Autodesk Inventor part; units mm, degrees
ref_plane "Work Plane1" through (0, 5, 0) normal (0, 1, 0) x (-1, 0, 0)
ref_plane "YZ Plane" through (0, 0, 0) normal (1, 0, 0) x (0, 1, 0)
ref_plane "XY Plane" through (0, 0, 0) normal (0, 0, 1) x (1, 0, 0)
sketch "Sketch1" plane through (0, 0, 0) normal (1, 0, 0) x (0, 1, 0)
  circle A0 centre (0, 0) radius 3.625
  circle A1 centre (0, 0) radius 5
  dimension "d0" = 7.25
  dimension "d1" = 10
extrude "Extrusion1" add sketch "Sketch1" along normal mid plane 20
ref_plane "Work Plane1" through (0, 5, 0) normal (0, 1, 0) x (-1, 0, 0)
sketch "Sketch2" plane through (0, 5, 0) normal (0, 1, 0) x (-1, 0, 0)
  line L0 (-1.65, 2.15) -> (1.65, 2.15)
  line L1 (1.65, 2.15) -> (1.65, -2.15)
  line L2 (1.65, -2.15) -> (-1.65, -2.15)
  line L3 (-1.65, -2.15) -> (-1.65, 2.15)
  line L4 (-1.65, 2.15) -> (1.65, -2.15) construction
  line L5 (1.65, 2.15) -> (-1.65, -2.15) construction
  line L6 (-4, 3) -> (4, 3)
  line L7 (4, 3) -> (4, -3)
  line L8 (4, -3) -> (-4, -3)
  line L9 (-4, -3) -> (-4, 3)
  line L10 (-4, 3) -> (4, -3) construction
  line L11 (4, 3) -> (-4, -3) construction
  arc A0 (1.65, -2.15) -> (1.65, 2.15) centre (0.0168, 0) ccw
  arc A1 (-1.65, 2.15) -> (-1.65, -2.15) centre (-0.0168, 0) ccw
  point P0 (0, 0)
  dimension "d4" = 3.3
  dimension "d5" = 4.3
  dimension "d9" = 8
  dimension "d10" = 6
  dimension "d15" = 2.7
  dimension "d16" = 2.7
extrude "Extrusion2" add sketch "Sketch2" against normal blind 4.125 contours L0 L1 L2 L3 | L3 A1 | A0 L1 | L6 L7 L8 L9
extrude "Extrusion3" cut sketch "Sketch2" against normal up to surface (4.125 mm away) contours L0 L1 L2 L3 | L3 A1 | A0 L1
ref_plane "Work Plane2" through (0, -5, 0) normal (0, 1, 0) x (-1, 0, 0)
sketch "Sketch3" plane through (0, -5, 0) normal (0, 1, 0) x (-1, 0, 0)
  line L0 (10, 3.625) -> (10, -3.625)
  line L1 (-10, 5) -> (-10, -5)
  line L2 (10, 2) -> (-10, 2)
  line L3 (-10, 2) -> (-10, -2)
  line L4 (-10, -2) -> (10, -2)
  line L5 (10, -2) -> (10, 2)
  point P0 (0, 0)
  point P1 (0, 2)
  dimension "d17" = 4
  dimension "d18" = 2
extrude "Extrusion4" add sketch "Sketch3" along normal blind 1
properties part number "part_holder"
The model under review builds one solid part; all positions refer to its coordinate system, in mm. A direction names the side the tool comes from. Round coordinates to 2 decimals unless told otherwise and drop trailing zeros. Order: outer loops, then holes, each group sorted by start corner. A loop starts at its lowest first (then second) coordinate and runs counter-clockwise, first axis right, second up. Notation, with made-up numbers: (82, 62) -> (120, 62) arc R21 cw to (120, 92) -> close; hole circle Ø5 at (0.25, 43). An arc over 180 degrees is marked (long way). Write item = value, one per line. Start each with the question number.
Item 1: Consider section A-A on y = 0. Write out the cut boundary in (x, z) (3 decimals), plus the area to 3 significant figures.
Item 2: Consider section C-C on x = 1.25. Write out the cut boundary in (y, z) (3 decimals).
Item 3: For line 1 along Z through (x, y) = (0, 0) (3 decimals); line 2 along Y through (x, z) = (-6.75, 4); line 3 along Z through (x, y) = (-7, -1.5), list the stretches that pass through material, from the lowest coordinate up.
Item 4: Mouldability with a two-part tool opening along Y and no side actions: class faces 4 (the face through (-0.14, 1.569, 4.747)), 5 (the face through (-4, 4.7, -2.3)), 6 (the face through (4, 2, 0)) as released by +Y, released by -Y, zero draft, split by the parting line, or undercut.
Item 5: Consider section D-D on y = -3. Write out the cut boundary in (x, z), plus the area to 3 significant figures.
Item 6: Clearance check with flat-ended pins moving along their axes: pin 1 Ø0.5 at (x, y) = (-1.5, 4.5) entering from -Z; pin 2 Ø2 at (x, y) = (6.5, 1.5) entering from +Z; pin 3 Ø6 at (y, z) = (0, 0) entering from +X. State where each tip first meets the part, or that it passes through.
Item 7: For faces 1 (the face through (4, 4.7, 2.3)), 2 (the face through (0, 3, 2.15)), 3 (the face through (-0.1, 4.5, -3)), list the 3-axis set-ups (+Z, -Z, +X, -X, +Y, -Y) from which the entire face can be reached by the end or side of a thin tool; tool diameter is ignored.
Item 8: Consider section B-B on x = 7.25. Write out the cut boundary in (y, z) (3 decimals), plus the area to 3 significant figures.
Conclusion:
q1.outline = (-10, -5) -> (10, -5) -> (10, -3.625) -> (-10, -3.625) -> close; (-10, 3.625) -> (10, 3.625) -> (10, 5) -> (-10, 5) -> close
q1.area = 55.0 mm2
q2.outline = (-5, -2) -> (-4.583, -2) arc R5 ccw to (4, -3) -> (5, -3) -> (5, -2.15) -> (0.875, -2.15) -> (0.875, -3) -> (2.035, -3) arc R3.625 cw (long way) to (2.035, 3) -> (0.875, 3) -> (0.875, 2.15) -> (5, 2.15) -> (5, 3) -> (4, 3) arc R5 ccw to (-4.583, 2) -> (-5, 2) -> close
q3.line_1 = -5 to -3.625, 3.625 to 5
q3.line_2 = -3 to 3
q3.line_3 = -4.77 to -3.3, 3.3 to 4.77
q4.face_4 = split by the parting line
q4.face_5 = zero draft
q4.face_6 = undercut
q5.outline = (-10, -4) -> (10, -4) -> (10, -2.03) -> (-10, -2.03) -> close; (-10, 2.03) -> (10, 2.03) -> (10, 4) -> (-10, 4) -> close
q5.area = 78.6 mm2
q6.pin_1 = -3
q6.pin_2 = 4.97
q6.pin_3 = 4
q7.face_1 = +Z, +X, +Y
q7.face_2 = +Y
q7.face_3 = -Z, +X, -X, +Y
q8.outline = (-5, -2) -> (-4.583, -2) arc R5 ccw (long way) to (-4.583, 2) -> (-5, 2) -> close; hole circle Ø7.25 at (0, 0)
q8.area = 37.8 mm2
